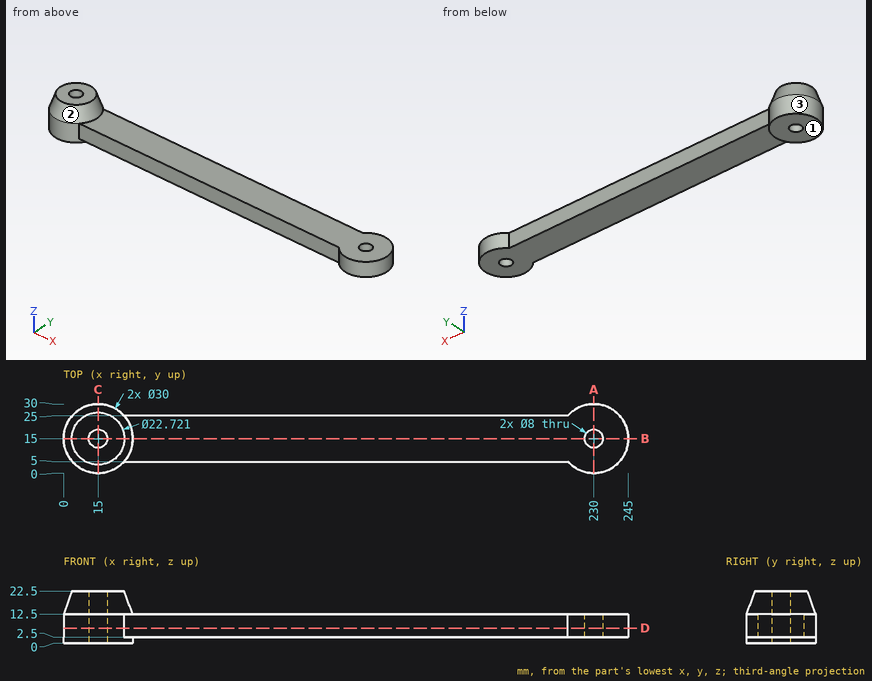
Geometry check sheet. Reference: drawing and pictorial views, mm from the part's lowest x, y, z. Give positions to 0.01 mm unless a question says otherwise; leave off trailing zeros. Loops run counter-clockwise (first coordinate to the right, second up) from the corner with the lowest first, then second, coordinate; pieces in that order, holes last. Notation, with made-up numbers: (54, 62.25) - (80, 62.25) arc R30 cw to (80, 86.25) - close; hole circle Ø9 at (19.5, -16.5). An arc over 180 degrees is marked (long way). One line per question, with ' | ' between items. Start each with the question number.
1. Draft check along X on the marked faces 1, 2 and 3. Enter one of: released by +X, released by -X, zero draft, split by the parting line, or undercut.
2. Cross-section at B-B, the plane y = 15. Enter the section's corners in (x, z).
3. Material ranges on line 1 along Y through (x, z) = (230, 7.25); line 2 along Z through (x, y) = (118, 20.75); line 3 along Y through (x, z) = (215, 3), recorded low to high. Write a range as [from, to].
4. Cross-section at C-C, the plane x = 15. Enter the section's corners in (y, z).
5. Cross-section at D-D, the plane z = 6.5. Enter the section's corners in (x, y).
6. Gauge pin test, flat ends, axial feed: pin 1 Ø12 at (x, z) = (219, 4.5) entering from +Y; pin 2 Ø9 at (x, y) = (96.5, 12) entering from -Z; pin 3 Ø5 at (y, z) = (4, 17) entering from -X (1 decimal); pin 4 Ø1.5 at (x, y) = (64.5, 4) entering from -Z. Record the tip position at first contact, or that the pin passes through.
7. Cross-section at A-A, the plane x = 230. Enter the section's corners in (y, z).
Check result:
1) face 1: zero draft | face 2: split by the parting line | face 3: undercut
2) outline: (0, 0) - (11, 0) - (11, 22.5) - (3.64, 22.5) - (0, 12.5) - close; (19, 0) - (30, 0) - (30, 2.5) - (226, 2.5) - (226, 12.5) - (30, 12.5) - (26.36, 22.5) - (19, 22.5) - close; (234, 2.5) - (245, 2.5) - (245, 12.5) - (234, 12.5) - close
3) line 1: y = [0, 11], [19, 30] | line 2: z = [2.5, 12.5] | line 3: y = [5, 25]
4) outline: (0, 0) - (11, 0) - (11, 22.5) - (3.64, 22.5) - (0, 12.5) - close; (19, 0) - (30, 0) - (30, 12.5) - (26.36, 22.5) - (19, 22.5) - close
5) outline: (26.18, 5) - (218.82, 5) arc R15 ccw (long way) to (218.82, 25) - (26.18, 25) arc R15 ccw (long way) to start; hole circle Ø8 at (15, 15); hole circle Ø8 at (230, 15)
6) pin 1: stops at y = 29.14 | pin 2: stops at z = 2.5 | pin 3: stops at x = 4.4 | pin 4: passes through
7) outline: (0, 2.5) - (11, 2.5) - (11, 12.5) - (0, 12.5) - close; (19, 2.5) - (30, 2.5) - (30, 12.5) - (19, 12.5) - close
